Design review of the part built by this model. Coordinates are the model's own, in mm. A direction names the side the tool comes from. Give positions to 0.01 mm unless a question says otherwise; leave off trailing zeros. Loops run counter-clockwise (first coordinate to the right, second up) from the corner with the lowest first, then second, coordinate; pieces in that order, holes last. Notation, with made-up numbers: (-35.75, 40) - (-20.75, 40) arc R32 cw to (-20.75, 67) - close; hole circle Ø4 at (55, 86). An arc over 180 degrees is marked (long way). Put each result on its own line as item: value. Start each with the question number.
```python
from build123d import *

# Parameters (mm, degrees)
CUT_EXTRUDE1_START  = 2.2987
CUT_EXTRUDE1_DEPTH  = 10.922
CIRPATTERN1_COUNT   = 10
BOSS_EXTRUDE1_START = -7.62
BOSS_EXTRUDE1_DEPTH = 7.62
CUT_EXTRUDE2_DEPTH  = 6.6802
BOSS_EXTRUDE2_START = 4.826
SKETCH8_R           = 11.1125
BOSS_EXTRUDE2_DEPTH = 4.826
CUT_EXTRUDE3_DEPTH  = 24.384
CHAMFER2_SIZE       = 0.5


with BuildPart() as part:
    # Sketch2 → Revolve1 (revolve)
    with BuildSketch(Plane(origin=(0, 0, 0), x_dir=(0, 0, -1), z_dir=(1, 0, 0)), mode=Mode.PRIVATE) as revolve1_sk:
        with BuildLine():
            Line((-3.9878, 2.5), (10.3124, 2.5))
            Line((10.3124, 2.5), (10.3124, 11.1125))
            Line((10.3124, 11.1125), (9.46785, 11.1125))
            ThreePointArc((9.46785, 11.1125), (8.846862309, 10.395787163), (8.6233, 9.4742))
            Line((8.6233, 9.4742), (8.6233, 7.8359))
            Line((8.6233, 7.8359), (-2.2987, 7.8359))
            Line((-2.2987, 7.8359), (-2.2987, 9.4742))
            ThreePointArc((-2.2987, 9.4742), (-2.522262309, 10.395787163), (-3.14325, 11.1125))
            Line((-3.14325, 11.1125), (-3.9878, 11.1125))
            Line((-3.9878, 11.1125), (-3.9878, 2.5))
        make_face()
    revolve(revolve1_sk.sketch.rotate(Axis((0, 0, 10.3124), (0, 0, -1)), 90), axis=Axis((0, 0, 10.3124), (0, 0, -1)))

    # Sketch3 → Cut-Extrude1 (cut)
    with BuildSketch(Plane.XY.offset(CUT_EXTRUDE1_START)):
        with BuildLine():
            Line((-0.635, 6.329348022), (0.635, 6.329348022))
            Line((0.635, 6.329348022), (1.287830721, 7.729348022))
            ThreePointArc((1.287830721, 7.729348022), (0, 7.8359), (-1.287830721, 7.729348022))
            Line((-1.287830721, 7.729348022), (-0.635, 6.329348022))
        make_face()
    cut_extrude1 = extrude(amount=-CUT_EXTRUDE1_DEPTH, mode=Mode.SUBTRACT)

    # CirPattern1: Cut-Extrude1 ×10 about axis
    cirpattern1_axis = Axis((0, 0, 0), (0, 0, 1))
    for i in range(1, CIRPATTERN1_COUNT):
        add(cut_extrude1.rotate(cirpattern1_axis, i * 360 / CIRPATTERN1_COUNT), mode=Mode.SUBTRACT)

    # Sketch5 → Boss-Extrude1 (add)
    with BuildSketch(Plane.XY.offset(3.9878).offset(BOSS_EXTRUDE1_START)):
        with BuildLine():
            Line((-2.291287847, 1), (2.291287847, 1))
            ThreePointArc((2.291287847, 1), (0, 2.5), (-2.291287847, 1))
        make_face()
    extrude(amount=BOSS_EXTRUDE1_DEPTH)

    # Sketch6 → Cut-Extrude2 (cut)
    with BuildSketch(Plane(origin=(0, 0, -10.3124), x_dir=(-1, 0, 0), z_dir=(0, 0, -1))):
        Polygon((5.672466395, 0), (2.836233197, 4.9125), (-2.836233197, 4.9125), (-5.672466395, 0), (-2.836233197, -4.9125), (2.836233197, -4.9125), align=None)
    extrude(amount=-CUT_EXTRUDE2_DEPTH, mode=Mode.SUBTRACT)

    # Sketch8 → Boss-Extrude2 (add)
    with BuildSketch(Plane.XY.offset(3.9878).offset(BOSS_EXTRUDE2_START)):
        Circle(SKETCH8_R)
        with BuildLine():
            Line((2.291287847, 1), (-2.291287847, 1))
            ThreePointArc((-2.291287847, 1), (0, -2.5), (2.291287847, 1))
        make_face(mode=Mode.SUBTRACT)
    extrude(amount=-BOSS_EXTRUDE2_DEPTH)

    # Sketch12 → Cut-Extrude3 (cut)
    with BuildSketch(Plane.XY.offset(8.8138)):
        with BuildLine():
            Line((2.479919354, 1.3), (-2.479919354, 1.3))
            ThreePointArc((-2.479919354, 1.3), (0, -2.8), (2.479919354, 1.3))
        make_face()
    extrude(amount=-CUT_EXTRUDE3_DEPTH, mode=Mode.SUBTRACT)

    # Chamfer2
    chamfer2_edges = [part.edges().sort_by_distance(p)[0] for p in [
        (-11.1125, 0, 8.8138),
        (0, -2.8, 8.8138),
        (0, 1.3, 8.8138),
    ]]
    chamfer(chamfer2_edges, length=CHAMFER2_SIZE)


solid = part.part
```
Item 1: Mouldability with a two-part tool opening along Y and no side actions: class faces 6 (the flat face through (0, 3, 8.814)), 7 (the flat face through (0, 6.329, -3)), 8 (the flat face through (3.71, 5.13, -3.09)) as pulls with the +Y half, pulls with the -Y half, needs draft (parallel to the pull), parting line crosses it, or undercut.
Item 2: Consider section A-A (x = 0). State the section outline as (y, z) points.
Item 3: Machinability: for faces 1 (the flat face through (0, 2, -3.632)), 2 (the cylindrical face through (-6.33, -4.62, -3.09)), 3 (the flat face through (6.4, 3.1, -3.1)), 4 (the flat face through (-0.957, -7.02, -3.086)), 5 (the cylindrical face through (-7.836, -0.016, -3.086)), which of the approach directions +Z, -Z, +X, -X, +Y, -Y give a long, thin tool a straight path to every point of the face, cutting with its end or side? Answer none if there is none.
Item 4: Consider section B-B (z = 6). State the section outline as (x, y) points (1 decimal).
Item 5: For P1, Ø3, axis at x = 0, z = -6.5, coming from the +Y side; P2, Ø8, axis at x = 0, y = -0.5, coming from the -Z side; P3, Ø0.6, axis at x = 0, z = -3.5, coming from the -Y side, all flat-tipped, find the tip position at first contact; note any pin that passes through.
Item 6: For L1, parallel to Z at x = -9, y = 0; L2, parallel to X at y = 0, z = -0.25; L3, parallel to Y at x = 0, z = 4.75, list the stretches that pass through material, from the lowest coordinate up. Write a range as from..to.
Geometry says:
1. face 6: needs draft
1. face 7: pulls with the +Y half
1. face 8: undercut
2. outline: (-11.11, -10.31) - (-4.91, -10.31) - (-4.91, -3.63) - (-2.8, -3.63) - (-2.8, 8.31) - (-3.3, 8.81) - (-10.61, 8.81) - (-11.11, 8.31) - (-11.11, 3.14) arc R2.01 ccw to (-9.47, 2.3) - (-6.33, 2.3) - (-6.33, -8.62) - (-9.47, -8.62) arc R2.01 ccw to (-11.11, -9.47) - close; (1.3, -3.63) - (4.91, -3.63) - (4.91, -10.31) - (11.11, -10.31) - (11.11, -9.47) arc R2.01 ccw to (9.47, -8.62) - (6.33, -8.62) - (6.33, 2.3) - (9.47, 2.3) arc R2.01 ccw to (11.11, 3.14) - (11.11, 8.31) - (10.61, 8.81) - (1.8, 8.81) - (1.3, 8.31) - close
3. face 1: -Z
3. face 2: -X, -Y
3. face 3: +X
3. face 4: -Y
3. face 5: -X
4. outline: circle Ø22.2 at (0, 0); hole (-2.5, 1.3) arc R2.8 ccw (long way) to (2.5, 1.3) - close
5. P1: stops at y = 7.73
5. P2: stops at z = -3.63
5. P3: stops at y = -6.33
6. L1: z = -10.31..-8.62, 2.3..8.81
6. L2: x = -7.84..-2.8, 2.8..7.84
6. L3: y = -11.11..-2.8, 1.3..11.11
